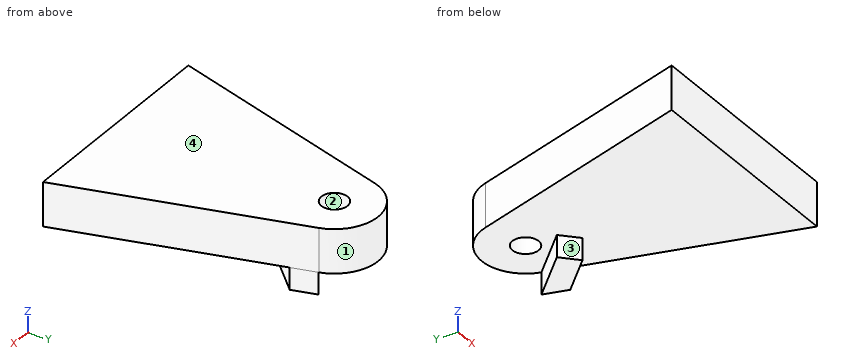
```python
from build123d import *

# Parameters (mm, degrees)
BOSS_EXTRUDE1_DEPTH = 2.54
BOSS_EXTRUDE2_DEPTH = 3.81
SKETCH3_R           = 0.762
CUT_EXTRUDE1_DEPTH  = 2.54


with BuildPart() as part:
    # Sketch1 → Boss-Extrude1 (new body)
    with BuildSketch(Plane.XY):
        with BuildLine():
            Line((-8.7884, 13.4112), (-12.7, 0))
            Line((-12.7, 0), (0, 0))
            Line((0, 0), (-3.9116, 13.4112))
            ThreePointArc((-3.9116, 13.4112), (-6.35, 15.24), (-8.7884, 13.4112))
        make_face()
    extrude(amount=BOSS_EXTRUDE1_DEPTH)

    # Sketch5 → Boss-Extrude2 (add)
    with BuildSketch(Plane.XY.offset(2.54)):
        Polygon((-6.318654584, 10.904222323), (-3.908374337, 13.400140584), (-3.498832415, 11.995996853), (-5.405093038, 10.022006193), align=None)
    extrude(amount=-BOSS_EXTRUDE2_DEPTH)

    # Sketch3 → Cut-Extrude1 (cut)
    with BuildSketch(Plane.XY.offset(2.54)):
        with Locations((-6.35, 12.7)):
            Circle(SKETCH3_R)
    extrude(amount=-CUT_EXTRUDE1_DEPTH, mode=Mode.SUBTRACT)


solid = part.part
```
Model file for the job. Use its own axes, mm. Face numbers are marked on the shaded views. Give positions to 0.01 mm unless a question says otherwise; leave off trailing zeros. Loops run counter-clockwise (first coordinate to the right, second up) from the corner with the lowest first, then second, coordinate; pieces in that order, holes last. Notation, with made-up numbers: (72, 5.25) -> (114, 5.25) arc R19 ccw to (114, 33.25) -> close; hole circle Ø10 at (-36, 5). An arc over 180 degrees is marked (long way). Write each question's results on one line, items separated by ' | '.
(1) Cut at B-B on y = 12.7. List the corners of the cut face in (x, z).
Geometry results:
outline: (-9, 0) -> (-7.11, 0) -> (-7.11, 2.54) -> (-9, 2.54) -> close; (-5.59, 0) -> (-4.58, 0) -> (-4.58, -1.27) -> (-3.7, -1.27) -> (-3.7, 2.54) -> (-5.59, 2.54) -> close
(2) Flat gauge pin, fed straight in: pin 1 Ø3 at (x, y) = (-8.5, 8) entering from -Z. Where does the tip first touch, or does it go through?
Geometry results:
pin 1: stops at z = 0
(3) Cut at D-D on z = -0.55. List the corners of the cut face in (x, y), and give its area (3 significant figures).
Geometry results:
outline: (-6.32, 10.9) -> (-5.41, 10.02) -> (-3.5, 12) -> (-3.91, 13.4) -> close | area: 3.95 mm²
(4) Cut at C-C on z = 0.8. List the corners of the cut face in (x, y), and give its area (3 significant figures).
Geometry results:
outline: (-12.7, 0) -> (0, 0) -> (-3.91, 13.41) arc R2.54 ccw to (-8.79, 13.41) -> close; hole circle Ø1.52 at (-6.35, 12.7) | area: 123 mm²
(5) Probe line 1 along Y through (x, z) = (-6.35, 1); line 2 along Z through (x, y) = (-4.25, 10); line 3 along Y through (x, z) = (-6.5, 1). List the from-to ranges inside material, lowest first.
Geometry results:
line 1: y = 0 to 11.94, 13.46 to 15.24 | line 2: z = 0 to 2.54 | line 3: y = 0 to 11.95, 13.45 to 15.24
(6) Pull direction Y, two halves, no side cores. Call the marked faces 1, 2, 3 and 4: released by +Y, released by -Y, zero draft, split by the parting line, or undercut.
Geometry results:
face 1: released by +Y | face 2: undercut | face 3: released by -Y | face 4: zero draft
(7) Cut at A-A on x = -6.5. List the corners of the cut face in (y, z), and give its area (3 significant figures).
Geometry results:
outline: (0, 0) -> (11.95, 0) -> (11.95, 2.54) -> (0, 2.54) -> close; (13.45, 0) -> (15.24, 0) -> (15.24, 2.54) -> (13.45, 2.54) -> close | area: 34.9 mm²
